The drawing under review shows one solid part. Ordinate dimensions are in mm from its lowest x, y, z. A direction names the side the tool comes from. Coordinates: 2 decimals unless noted, no trailing zeros. Order: outer loops, then holes, each group sorted by start corner. A loop starts at its lowest first (then second) coordinate and runs counter-clockwise, first axis right, second up.
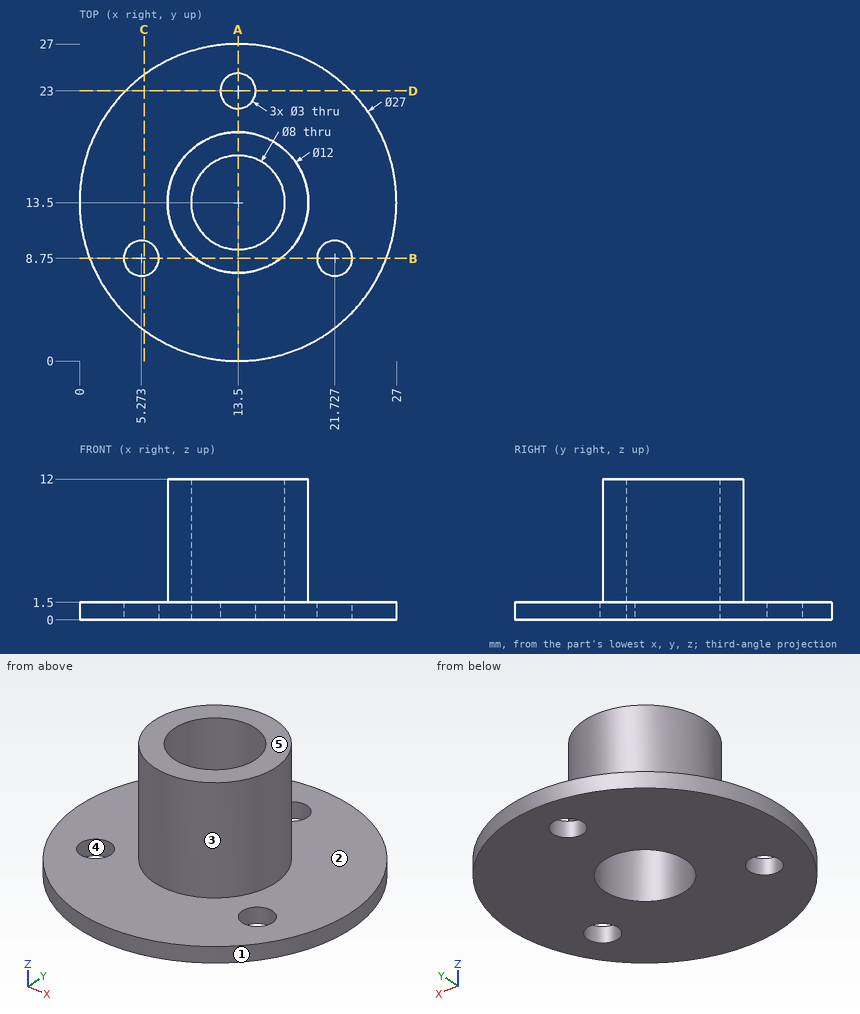
(1) Machinability: for the marked faces 1 and 2, which of the approach directions +Z, -Z, +X, -X, +Y, -Y give a long, thin tool a straight path to every point of the face, cutting with its end or side? Answer none if there is none.
A:
face 1: +Z, -Z
face 2: +Z
(2) For pin 1 Ø5 at (y, z) = (14, 7) entering from +X; pin 2 Ø2.5 at (x, y) = (5.27, 8.75) entering from -Z; pin 3 Ø3 at (x, z) = (14.5, 7.5) entering from -Y; pin 4 Ø6 at (x, z) = (17.5, 5) entering from -Y, all flat-tipped, find the tip position at first contact; note any pin that passes through.
A:
pin 1: stops at x = 19.5
pin 2: passes through
pin 3: stops at y = 7.5
pin 4: stops at y = 7.58
(3) We need section A-A, the plane x = 13.5. Write out the cut boundary in (y, z), and give its area (3 significant figures).
A:
outline: (0, 0) - (9.5, 0) - (9.5, 12) - (7.5, 12) - (7.5, 1.5) - (0, 1.5) - close; (17.5, 0) - (21.5, 0) - (21.5, 1.5) - (19.5, 1.5) - (19.5, 12) - (17.5, 12) - close; (24.5, 0) - (27, 0) - (27, 1.5) - (24.5, 1.5) - close
area: 66.0 mm2
(4) Draft analysis for pull direction X (two halves, no side actions). For the marked faces 3, 4 and 5, state which applies: released by +X, released by -X, zero draft, split by the parting line, or undercut.
A:
face 3: split by the parting line
face 4: undercut
face 5: zero draft
(5) We need section B-B, the plane y = 8.75. Write out the cut boundary in (x, z), and give its area (3 significant figures).
A:
outline: (0.86, 0) - (3.77, 0) - (3.77, 1.5) - (0.86, 1.5) - close; (6.77, 0) - (20.23, 0) - (20.23, 1.5) - (17.17, 1.5) - (17.17, 12) - (9.83, 12) - (9.83, 1.5) - (6.77, 1.5) - close; (23.23, 0) - (26.14, 0) - (26.14, 1.5) - (23.23, 1.5) - close
area: 106 mm2
(6) Wall thickness on probe 1 along Y at (x, z) = (13.5, 0.85); probe 2 along Y at (x, z) = (10.25, 9) (1 decimal); probe 3 along Z at (x, y) = (16, 3.75): over which ranges is each line inside the solid? List them lowest first.
A:
probe 1: y = 0 to 9.5, 17.5 to 21.5, 24.5 to 27
probe 2: y = 8.5 to 11.2, 15.8 to 18.5
probe 3: z = 0 to 1.5
(7) We need section D-D, the plane y = 23. Write out the cut boundary in (x, z), and give its area (3 significant figures).
A:
outline: (3.91, 0) - (12, 0) - (12, 1.5) - (3.91, 1.5) - close; (15, 0) - (23.09, 0) - (23.09, 1.5) - (15, 1.5) - close
area: 24.3 mm2
(8) We need section C-C, the plane x = 5.5. Write out the cut boundary in (y, z).
A:
outline: (2.63, 0) - (7.27, 0) - (7.27, 1.5) - (2.63, 1.5) - close; (10.23, 0) - (24.37, 0) - (24.37, 1.5) - (10.23, 1.5) - close
